Autodesk Inventor part; units mm, degrees
ref_plane "YZ Plane" through (0, 0, 0) normal (1, 0, 0) x (0, 1, 0)
ref_plane "XZ Plane" through (0, 0, 0) normal (0, 1, 0) x (-1, 0, 0)
ref_plane "XY Plane" through (0, 0, 0) normal (0, 0, 1) x (1, 0, 0)
sketch "Sketch1" plane through (0, 0, 0) normal (0, 1, 0) x (-1, 0, 0)
  line L0 (-14, -14) -> (14, -14)
  line L1 (14, -14) -> (14, 14)
  line L2 (14, 14) -> (-14, 14)
  line L3 (-14, 14) -> (-14, -14)
  line L4 (-14, -14) -> (14, 14) construction
  line L5 (14, -14) -> (-14, 14) construction
  point P0 (0, 0)
  dimension "d0" = 28
  dimension "d1" = 28
extrude "Extrusion1" add sketch "Sketch1" against normal blind 3
hole "Hole1" at (0, 0, 0) direction (0, -1, 0) diameter 5 end through all countersink diameter 7.5 countersink angle 90
fillet "Fillet1" radius 1 4 edges at (14, -1.5, 14) (14, -1.5, -14) (-14, -1.5, -14) (-14, -1.5, 14)
fillet "Fillet2" radius 0.3 16 edges at (13.7071, 0, 13.7071) (14, 0, 0) (13.7071, 0, -13.7071) (0, 0, -14) (-13.7071, 0, -13.7071) (-14, 0, 0) (-13.7071, 0, 13.7071) (0, 0, 14) (-13.7071, -3, 13.7071) (-14, -3, 0) (-13.7071, -3, -13.7071) (0, -3, -14) (13.7071, -3, -13.7071) (14, -3, 0) (13.7071, -3, 13.7071) (0, -3, 14)
properties part number "clampPlate" material "Steel, High Strength, Low Alloy"
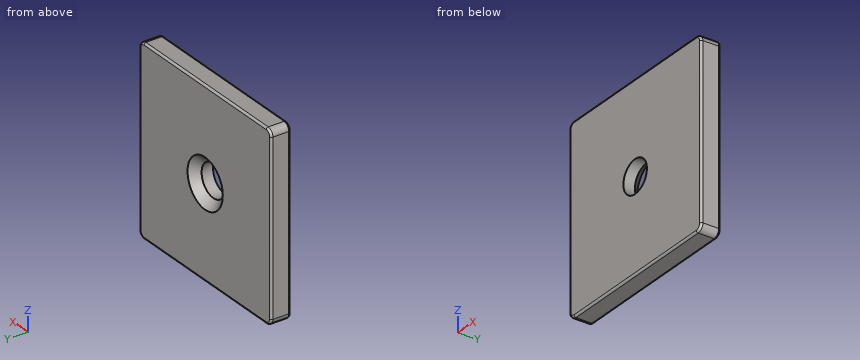
Geometry: final body of the model. Coordinates: model frame, mm. Round coordinates to 2 decimals unless told otherwise and drop trailing zeros. Write each loop counter-clockwise with the first axis right and the second up, starting at its lowest first coordinate (ties: lowest second). Pieces come first, ordered by that corner, then holes. Notation, with made-up numbers: M -22,40.5 L 0,40.5 A30 cw 0,69.5 Z; hole C -15.75,13.5 d11. An arc over 180 degrees is marked long. Answer in a Markdown table with one row per item. Add a question column.
(1) Cut plane C-C, the plane z = 0. Return the cut outline in (x, y).
(2) Cut plane A-A, the plane y = -0.8. Return the cut outline in (x, z), then the cut area to 3 significant figures.
(3) Contact query for a flat-ended pin moving along its axis: pin 1 (6 mm diameter, centred on x = 0, z = 0, fed in from +Y). Output: stop coordinate, or through.
(4) Ray query, L1, parallel to X at y = -2.2, z = 0; L2, parallel to Z at x = -2.5, y = -0.3. Return the intervals inside material, ascending.
(5) Cut plane B-B, the plane x = 0. Return the cut outline in (y, z).
(6) Cut plane D-D, the plane y = -2.35. Return the cut outline in (x, z), then the cut area to 3 significant figures.
Established:
| question | item | result |
|---|---|---|
| 1 | outline | M -14,-2.7 A0.3 ccw -13.7,-3 L -2.5,-3 L -2.5,-1.25 L -3.75,0 L -13.7,0 A0.3 ccw -14,-0.3 Z; M 2.5,-3 L 13.7,-3 A0.3 ccw 14,-2.7 L 14,-0.3 A0.3 ccw 13.7,0 L 3.75,0 L 2.5,-1.25 Z |
| 2 | outline | M -14,-13 A1 ccw -13,-14 L 13,-14 A1 ccw 14,-13 L 14,13 A1 ccw 13,14 L -13,14 A1 ccw -14,13 Z; hole C 0,0 d5.9 |
| 2 | area | 756 mm² |
| 3 | pin 1 | y = -0.75 |
| 4 | L1 | -14 to -2.5, 2.5 to 14 |
| 4 | L2 | -14 to -2.38, 2.38 to 14 |
| 5 | outline | M -3,-13.7 A0.3 ccw -2.7,-14 L -0.3,-14 A0.3 ccw 0,-13.7 L 0,-3.75 L -1.25,-2.5 L -3,-2.5 Z; M -3,2.5 L -1.25,2.5 L 0,3.75 L 0,13.7 A0.3 ccw -0.3,14 L -2.7,14 A0.3 ccw -3,13.7 Z |
| 6 | outline | M -14,-13 A1 ccw -13,-14 L 13,-14 A1 ccw 14,-13 L 14,13 A1 ccw 13,14 L -13,14 A1 ccw -14,13 Z; hole C 0,0 d5 |
| 6 | area | 764 mm² |
